Build history of the part. All positions in model axes, mm. Face numbers are marked on the shaded views. Coordinates: 2 decimals unless noted, no trailing zeros. Loops run counter-clockwise (first coordinate to the right, second up) from the corner with the lowest first, then second, coordinate; pieces in that order, holes last.
(1) Wall check: L1, parallel to Y at x = -10.75, z = 10 (3 decimals); L2, parallel to Z at x = -2, y = 17.5; L3, parallel to X at y = 19.5, z = 5.25. Give the ranges that are in metal, low to high.
(2) Slice it at C-C (z = 7.25). Give the cut face in (x, y), and give its area (3 significant figures).
(3) Flat gauge pins, fed straight in: P1, Ø3, axis at x = -20, y = 11.5, coming from the +Z side; P2, Ø3, axis at x = -11.5, z = 9, coming from the -Y side; P3, Ø7.5, axis at x = -18.5, y = -1.5, coming from the +Z side. Where does each tip first touch, or does it go through?
(4) Two-plate mould, pull along X, no slides. Class the marked faces 1, 2 and 3: pulls with the +X half, pulls with the -X half, needs draft (parallel to the pull), parting line crosses it, or undercut.
(5) Slice it at A-A (z = 4.75). Give the cut face in (x, y), and give its area (3 significant figures).
(6) Slice it at D-D (x = -7.25). Give the cut face in (y, z).
(7) Slice it at B-B (y = -16.5). Give the cut face in (x, z).
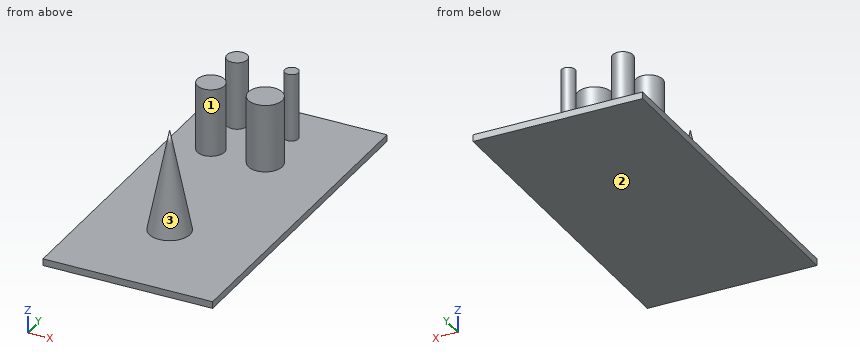
from build123d import *

# Parameters (mm, degrees)
F0_W     = 50
F0_H     = 50
F1_DEPTH = 1
F2_R     = 1.5
F2_R_2   = 1
F2_R_3   = 2
F2_R_4   = 2.5
F3_DEPTH = 10
F4_R     = 3
F8_W     = 25
F8_H     = 50
F9_DEPTH = 1


with BuildPart() as f1:
    # F0 (on Top) → F1 (new body)
    with BuildSketch(Plane.XY):
        Rectangle(F0_W, F0_H)
    extrude(amount=F1_DEPTH)

    # F2 (on face) → F3 (join)
    with BuildSketch(Plane.XY.offset(1)):
        with Locations((-18.8301634043, 18.6664275825)):
            Circle(F2_R)
        with Locations((-10.8068743721, 18.6664275825)):
            Circle(F2_R_2)
        with Locations((-18.8301634043, 11.1343609169)):
            Circle(F2_R_3)
        with Locations((-10.8068743721, 11.1343609169)):
            Circle(F2_R_4)
    extrude(amount=F3_DEPTH)

    # F4 (on face) → F7 section 0
    with BuildSketch(Plane.XY.offset(1), mode=Mode.PRIVATE) as f7_s0:
        with Locations((-13.8089349493, -10.4548223317)):
            Circle(F4_R)
    loft([f7_s0.sketch, Vertex(-13.8089349493, -10.4548223317, 16)])

    # F8 (on face) → F9 (cut, through all)
    with BuildSketch(Plane.XY.offset(1)):
        with Locations((12.5, 0)):
            Rectangle(F8_W, F8_H)
    extrude(amount=-F9_DEPTH, mode=Mode.SUBTRACT)


solid = f1.part
Response values:
1. L1: y = 8.635 to 13.634, 17.668 to 19.665
1. L2: z = 0 to 1
1. L3: x = -20.08 to -17.58, -11.36 to -10.25
2. outline: circle Ø4 at (-18.83, 11.13); circle Ø3 at (-18.83, 18.67); circle Ø3.5 at (-13.81, -10.45); circle Ø5 at (-10.81, 11.13); circle Ø2 at (-10.81, 18.67)
2. area: 52.0 mm2
3. P1: stops at z = 11
3. P2: stops at y = -11.66
3. P3: stops at z = 1
4. face 1: undercut
4. face 2: needs draft
4. face 3: parting line crosses it
5. outline: circle Ø4 at (-18.83, 11.13); circle Ø3 at (-18.83, 18.67); circle Ø4.5 at (-13.81, -10.45); circle Ø5 at (-10.81, 11.13); circle Ø2 at (-10.81, 18.67)
5. area: 58.3 mm2
6. outline: (-25, 0) - (25, 0) - (25, 1) - (-25, 1) - close
7. outline: (-25, 0) - (0, 0) - (0, 1) - (-25, 1) - close
